Job drawing, mm, ordinate dimensions from the low corner. One solid piece. A direction names the side the tool comes from. Coordinates: 2 decimals unless noted, no trailing zeros. Loops run counter-clockwise (first coordinate to the right, second up) from the corner with the lowest first, then second, coordinate; pieces in that order, holes last. Notation, with made-up numbers: (62, -8.75) -> (116, -8.75) arc R27 cw to (116, 23.25) -> close; hole circle Ø6 at (59.5, 84). An arc over 180 degrees is marked (long way). Use one line per item in the form item = value. Start each with the question number.
(1) 3-axis set-ups, long thin cutter, end or side, ignore diameter. For the marked faces 1, 2 and 3: which of +Z, -Z, +X, -X, +Y, -Y reach the whole face in a straight line?
(2) Band-saw the part on C-C on z = 8. Give the cut face in (x, y), then the cut area to 3 significant figures.
(3) Mould opens along Y. For the marked faces 4, 5, 6 and 7 say: +Y half, -Y half, draft (parallel to the pull), parting line (faces both ways), or undercut.
(4) Drill centre lines: L1, parallel to Y at x = 60, z = 4; L2, parallel to Y at x = 14, z = 6; L3, parallel to Y at x = 30, z = 13.5. Where is each one in solid material? Low to high. Write a range as [from, to].
(5) Pin check, flat tips, straight feed: P1, Ø5, axis at y = 12.5, z = 5.5, coming from the +X side; P2, Ø5, axis at y = 14, z = 5, coming from the -X side; P3, Ø5, axis at x = 21.5, z = 11, coming from the -Y side; P4, Ø6, axis at x = 73.5, y = 12, coming from the -Z side. Stop position of each tip, or through.
(6) Band-saw the part on B-B on y = 32.5. Give the cut face in (x, z), then the cut area to 3 significant figures.
(7) Band-saw the part on A-A on x = 60. Give the cut face in (y, z).
(8) Band-saw the part on D-D on x = 22.5. Give the cut face in (y, z), then the cut area to 3 significant figures.
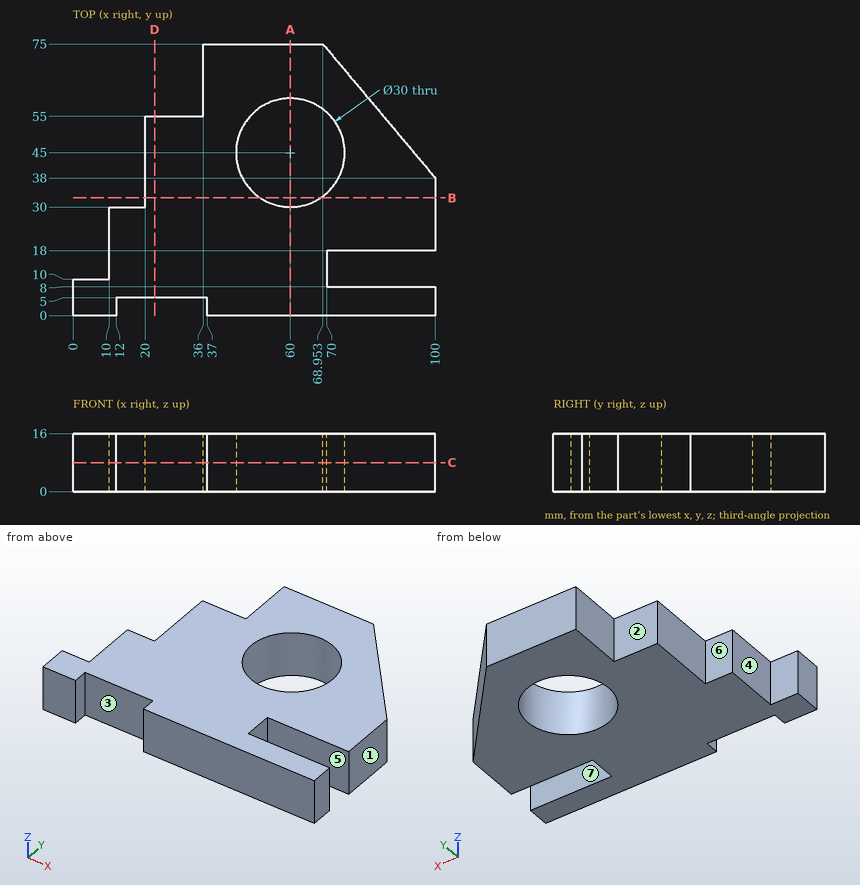
A:
q1.face_1 = +Z, -Z, +X, +Y, -Y
q1.face_2 = +Z, -Z, -X, +Y
q1.face_3 = +Z, -Z, -Y
q2.outline = (0, 0) -> (12, 0) -> (12, 5) -> (37, 5) -> (37, 0) -> (100, 0) -> (100, 8) -> (70, 8) -> (70, 18) -> (100, 18) -> (100, 38) -> (68.95, 75) -> (36, 75) -> (36, 55) -> (20, 55) -> (20, 30) -> (10, 30) -> (10, 10) -> (0, 10) -> close; hole circle Ø30 at (60, 45)
q2.area = 4,370 mm²
q3.face_4 = draft
q3.face_5 = undercut
q3.face_6 = +Y half
q3.face_7 = undercut
q4.L1 = [0, 30], [60, 75]
q4.L2 = [5, 30]
q4.L3 = [5, 55]
q5.P1 = 70
q5.P2 = 10
q5.P3 = 5
q5.P4 = through
q6.outline = (20, 0) -> (51.71, 0) -> (51.71, 16) -> (20, 16) -> close; (68.29, 0) -> (100, 0) -> (100, 16) -> (68.29, 16) -> close
q6.area = 1,010 mm²
q7.outline = (0, 0) -> (30, 0) -> (30, 16) -> (0, 16) -> close; (60, 0) -> (75, 0) -> (75, 16) -> (60, 16) -> close
q8.outline = (5, 0) -> (55, 0) -> (55, 16) -> (5, 16) -> close
q8.area = 800 mm²
